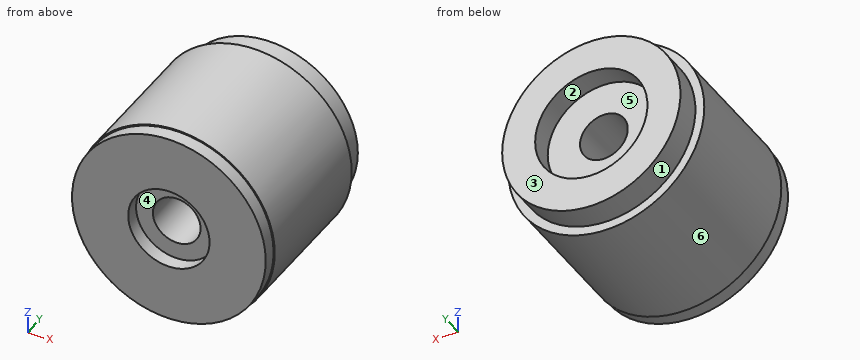
from build123d import *

# Parameters (mm, degrees)
SKETCH1_R           = 34.91
BOSS_EXTRUDE1_DEPTH = 63.5
SKETCH2_OUTSIDE_W   = 95.3
SKETCH2_OUTSIDE_H   = 95.3
SKETCH2_OUTSIDE_R   = 34.5
CUT_EXTRUDE1_DEPTH  = 5
SKETCH3_OUTSIDE_W   = 95.3
SKETCH3_OUTSIDE_H   = 95.3
SKETCH3_OUTSIDE_R   = 31.75
CUT_EXTRUDE2_DEPTH  = 9.52
SKETCH4_R           = 20
CUT_EXTRUDE3_DEPTH  = 8
SKETCH5_R           = 8.5
CUT_EXTRUDE4_DEPTH  = 64.5
SKETCH6_R           = 14.5
CUT_EXTRUDE5_DEPTH  = 5


with BuildPart() as part:
    # Sketch1 → Boss-Extrude1 (new body)
    with BuildSketch(Plane(origin=(0, 0, 0), x_dir=(1, 0, 0), z_dir=(0, 1, 0))):
        Circle(SKETCH1_R)
    extrude(amount=BOSS_EXTRUDE1_DEPTH)

    # Sketch2 outside → Cut-Extrude1 (cut)
    with BuildSketch(Plane.XZ):
        Rectangle(SKETCH2_OUTSIDE_W, SKETCH2_OUTSIDE_H)
        Circle(SKETCH2_OUTSIDE_R, mode=Mode.SUBTRACT)
    extrude(amount=-CUT_EXTRUDE1_DEPTH, mode=Mode.SUBTRACT)

    # Sketch3 outside → Cut-Extrude2 (cut)
    with BuildSketch(Plane(origin=(0, 63.5, 0), x_dir=(1, 0, 0), z_dir=(0, 1, 0))):
        Rectangle(SKETCH3_OUTSIDE_W, SKETCH3_OUTSIDE_H)
        Circle(SKETCH3_OUTSIDE_R, mode=Mode.SUBTRACT)
    extrude(amount=-CUT_EXTRUDE2_DEPTH, mode=Mode.SUBTRACT)

    # Sketch4 → Cut-Extrude3 (cut)
    with BuildSketch(Plane(origin=(0, 63.5, 0), x_dir=(1, 0, 0), z_dir=(0, 1, 0))):
        Circle(SKETCH4_R)
    extrude(amount=-CUT_EXTRUDE3_DEPTH, mode=Mode.SUBTRACT)

    # Sketch5 → Cut-Extrude4 (cut, through all)
    with BuildSketch(Plane.XZ):
        Circle(SKETCH5_R)
    extrude(amount=-CUT_EXTRUDE4_DEPTH, mode=Mode.SUBTRACT)

    # Sketch6 → Cut-Extrude5 (cut)
    with BuildSketch(Plane.XZ):
        Circle(SKETCH6_R)
    extrude(amount=-CUT_EXTRUDE5_DEPTH, mode=Mode.SUBTRACT)


solid = part.part
Can you work these out from the model? Positions are in its coordinate system, mm. Face numbers are marked on the shaded views. A direction names the side the tool comes from. Coordinates: 2 decimals unless noted, no trailing zeros. Loops run counter-clockwise (first coordinate to the right, second up) from the corner with the lowest first, then second, coordinate; pieces in that order, holes last. Notation, with made-up numbers: M 87,-16 L 122,-16 A19 cw 122,16 Z; hole C 86.5,57.25 d2. An arc over 180 degrees is marked long. Return JSON: item names as keys, results as strings. Group by question number.
Item 1: Imagine slicing it at B-B (z = 0). Please give me the cut outline in (x, y), and give its area (3 significant figures).
Item 2: Imagine slicing it at A-A (x = 0). Please give me the cut outline in (y, z).
Item 3: If I drill on L1, parallel to Z at x = 0, y = 19; L2, parallel to Z at x = 0, y = 2; L3, parallel to Y at x = -7, z = -6, over which ranges is the centre line in solid material (lowest first)? Write a range as from..to.
Item 4: Thinking about a two-plate mould opening in X: for the marked faces 1, 2, 3 and 4, which applies, released by +X, released by -X, zero draft, split by the parting line, or undercut?
Item 5: On a 3-axis mill with a long thin cutter (end or side, diameter ignored), from which of +Z, -Z, +X, -X, +Y, -Y can I reach the whole of each face in a straight line? I mean the marked faces 5 and 6. Say none if no direction works.
Item 6: I'm going to push flat-ended pins straight in: pin 1 Ø2 at (y, z) = (24.5, -7) entering from +X; pin 2 Ø1.5 at (y, z) = (6.5, -6.5) entering from -X; pin 3 Ø1.5 at (x, y) = (-10, 55.5) entering from -Z. Where does each tip first touch, or does it pass through?
Item 7: Imagine slicing it at C-C (x = -16). Please give me the cut outline in (y, z), and give its area (3 significant figures).
Item 8: Imagine slicing it at D-D (y = 51). Please give me the cut outline in (x, z), and give its area (3 significant figures).
Verdict:
{
 "1": {"outline": "M -34.91,5 L -34.5,5 L -34.5,0 L -14.5,0 L -14.5,5 L -8.5,5 L -8.5,55.5 L -20,55.5 L -20,63.5 L -31.75,63.5 L -31.75,53.98 L -34.91,53.98 Z; M 8.5,5 L 14.5,5 L 14.5,0 L 34.5,0 L 34.5,5 L 34.91,5 L 34.91,53.98 L 31.75,53.98 L 31.75,63.5 L 20,63.5 L 20,55.5 L 8.5,55.5 Z", "area": "3,050 mm^2"},
 "2": {"outline": "M 0,-34.5 L 5,-34.5 L 5,-34.91 L 53.98,-34.91 L 53.98,-31.75 L 63.5,-31.75 L 63.5,-20 L 55.5,-20 L 55.5,-8.5 L 5,-8.5 L 5,-14.5 L 0,-14.5 Z; M 0,14.5 L 5,14.5 L 5,8.5 L 55.5,8.5 L 55.5,20 L 63.5,20 L 63.5,31.75 L 53.98,31.75 L 53.98,34.91 L 5,34.91 L 5,34.5 L 0,34.5 Z"},
 "3": {"L1": "z = -34.91..-8.5, 8.5..34.91", "L2": "z = -34.5..-14.5, 14.5..34.5", "L3": "y = 5..55.5"},
 "4": {"face 1": "split by the parting line", "face 2": "undercut", "face 3": "zero draft", "face 4": "undercut"},
 "5": {"face 5": "+Y", "face 6": "+Y, -Y"},
 "6": {"pin 1": "stops at x = 34.39", "pin 2": "stops at x = -34.43", "pin 3": "stops at z = -30.37"},
 "7": {"outline": "M 0,-30.57 L 5,-30.57 L 5,-31.03 L 53.98,-31.03 L 53.98,-27.42 L 63.5,-27.42 L 63.5,-12 L 55.5,-12 L 55.5,12 L 63.5,12 L 63.5,27.42 L 53.98,27.42 L 53.98,31.03 L 5,31.03 L 5,30.57 L 0,30.57 Z", "area": "3,680 mm^2"},
 "8": {"outline": "C 0,0 d69.82; hole C 0,0 d17", "area": "3,600 mm^2"}
}
